Can you work these out from the model? Positions are in its coordinate system, mm. A direction names the side the tool comes from. Round coordinates to 2 decimals unless told otherwise and drop trailing zeros. Write each loop counter-clockwise with the first axis right and the second up, starting at its lowest first coordinate (ties: lowest second). Pieces come first, ordered by that corner, then holes. Notation, with made-up numbers: (2.5, -35.5) -> (53.5, -35.5) arc R37 cw to (53.5, 0.5) -> close; hole circle Ø6 at (73, 14). An arc over 180 degrees is marked (long way). Write item = value, one per line. Start each with the question number.
1) Imagine slicing it at C-C, the plane y = 12.25. Please give me the cut outline in (x, z), then the cut area to 3 significant figures.
2) Thinking about a two-plate mould opening in X: for faces 4 (the face through (25, 1, -17)), 5 (the face through (-12.97, 10.39, -18.84)), 6 (the face through (0, 3, 20)), 7 (the face through (-25, 1, -17)), which applies, +X half, -X half, draft (parallel to the pull), parting line (faces both ways), or undercut?
3) For faces 1 (the face through (20, 1, -12)), 2 (the face through (0, 1, 18)), 3 (the face through (-20, 1, 12)), which set-ups out of +Z, -Z, +X, -X, +Y, -Y let a thin tool reach every point of the face, with its end or its side?
4) If I drill on line 1 (X direction, y = 1.6, z = 16.5); line 2 (X direction, y = 0.75, z = -16.5); line 3 (X direction, y = 2.5, z = -11), over which ranges is the centre line in solid material (lowest first)?
5) I'm going to push flat-ended pins straight in: pin 1 (7 mm diameter, centred on x = -1, z = -15, fed in from +Y); pin 2 (2 mm diameter, centred on y = 5.5, z = 1, fed in from -X); pin 3 (5.5 mm diameter, centred on y = 15, z = 12, fed in from +X). Where does each tip first touch, or does it pass through?
6) Imagine slicing it at B-B, the plane z = -7.5. Please give me the cut outline in (x, y).
7) Imagine slicing it at D-D, the plane x = 14. Please give me the cut outline in (y, z).
8) Imagine slicing it at A-A, the plane x = -20. Please give me the cut outline in (y, z), then the cut area to 3 significant figures.
from build123d import *

# Parameters (mm, degrees)
ESBO_O1_W                  = 30
ESBO_O1_H                  = 50
ESBO_O1_W_2                = 22
ESBO_O1_H_2                = 42
RESSALTO_EXTRUS_O1_DEPTH   = 20
ESBO_O3_R                  = 1.75
CORTE_EXTRUS_O2_DEPTH      = 44.874821937
CORTE_EXTRUS_O3_DEPTH      = 44.874821937
CORTE_EXTRUS_O3_DEPTH_BACK = 44.874821937
ESBO_O6_R                  = 1.75
ESBO_O6_W                  = 50
ESBO_O6_H                  = 9
RESSALTO_EXTRUS_O2_DEPTH   = 3


with BuildPart() as part:
    # Esbo_o1 → Ressalto-extrus_o1 (new body)
    with BuildSketch(Plane(origin=(0, 0, 0), x_dir=(1, 0, 0), z_dir=(0, 1, 0))):
        Rectangle(ESBO_O1_W, ESBO_O1_H)
        Rectangle(ESBO_O1_W_2, ESBO_O1_H_2, mode=Mode.SUBTRACT)
    extrude(amount=RESSALTO_EXTRUS_O1_DEPTH)

    # Esbo_o3 → Corte-extrus_o2 (cut, through all)
    with BuildSketch(Plane(origin=(15, 0, 0), x_dir=(0, 0, -1), z_dir=(1, 0, 0))):
        with Locations((-12, 15)):
            Circle(ESBO_O3_R)
        with Locations((12, 15)):
            Circle(ESBO_O3_R)
    extrude(amount=-CORTE_EXTRUS_O2_DEPTH, mode=Mode.SUBTRACT)

    # Esbo_o5 → Corte-extrus_o3 (cut, two sides: drawn at the far end of the back side and taken through both)
    with BuildSketch(Plane.ZY.offset(15).offset(-CORTE_EXTRUS_O3_DEPTH_BACK)):
        with BuildLine():
            Line((-16.736274298, 16.602406244), (-21, 4))
            Line((-21, 4), (-21, 0))
            Line((-21, 0), (-25, 0))
            Line((-25, 0), (-25, 4))
            Line((-25, 4), (-25, 20))
            Line((-25, 20), (-12, 20))
            ThreePointArc((-12, 20), (-14.914444096, 19.062759605), (-16.736274298, 16.602406244))
        make_face()
        with BuildLine():
            Line((25, 0), (25, 4))
            Line((25, 4), (25, 20))
            Line((25, 20), (12, 20))
            ThreePointArc((12, 20), (14.914444096, 19.062759605), (16.736274298, 16.602406244))
            Line((16.736274298, 16.602406244), (21, 4))
            Line((21, 4), (21, 0))
            Line((21, 0), (25, 0))
        make_face()
    extrude(amount=CORTE_EXTRUS_O3_DEPTH + CORTE_EXTRUS_O3_DEPTH_BACK, mode=Mode.SUBTRACT)


with BuildPart() as corte_extrus_o3_piece_1:
    # of the separate pieces the step leaves, piece 1, a body of its own (corte_extrus_o3_pieces)
    add(part.part.solids().sort_by_distance((-15, 0, 21))[0])



with BuildPart() as corte_extrus_o3_piece_2:
    # of the separate pieces the step leaves, piece 2, a body of its own (corte_extrus_o3_pieces)
    add(part.part.solids().sort_by_distance((15, 0, -21))[0])


with BuildPart() as corte_extrus_o3_piece_1_1:
    add(corte_extrus_o3_piece_1.part)

    add(corte_extrus_o3_piece_2.part)  # Ressalto-extrus_o2 merges Corte-extrus_o3 piece 2
    # Esbo_o6 → Ressalto-extrus_o2 (add)
    # profile 1 of 2: a face of its own
    with BuildSketch(Plane.XZ):
        Polygon((-15, 21), (15, 21), (25, 21), (25, 12), (15, 12), (15, 18), (-15, 18), (-15, 12), (-25, 12), (-25, 21), align=None)
        with Locations(Location((20, 16.5, 0), (0, 0, 90))):
            Circle(ESBO_O6_R, mode=Mode.SUBTRACT)
        with Locations(Location((-20, 16.5, 0), (0, 0, 90))):
            Circle(ESBO_O6_R, mode=Mode.SUBTRACT)
    # profile 2 of 2: a face of its own
    with BuildSketch(Plane.XZ):
        with Locations((0, -16.5)):
            Rectangle(ESBO_O6_W, ESBO_O6_H)
        with Locations(Location((-20, -16.5, 0), (0, 0, 270))):
            Circle(ESBO_O6_R, mode=Mode.SUBTRACT)
        with Locations(Location((20, -16.5, 0), (0, 0, 270))):
            Circle(ESBO_O6_R, mode=Mode.SUBTRACT)
    extrude(amount=-RESSALTO_EXTRUS_O2_DEPTH)


solid = corte_extrus_o3_piece_1_1.part
Reported:
q1.outline = (-15, -18.21) -> (-11, -18.21) -> (-11, 18.21) -> (-15, 18.21) -> close; (11, -18.21) -> (15, -18.21) -> (15, 18.21) -> (11, 18.21) -> close
q1.area = 291 mm²
q2.face_4 = +X half
q2.face_5 = draft
q2.face_6 = undercut
q2.face_7 = -X half
q3.face_1 = +X, +Y, -Y
q3.face_2 = +Y, -Y
q3.face_3 = -X, +Y, -Y
q4.line_1 = -25 to -21.75, -18.25 to -11, 11 to 18.25, 21.75 to 25
q4.line_2 = -25 to -21.75, -18.25 to 18.25, 21.75 to 25
q4.line_3 = -15 to -11, 11 to 15
q5.pin_1 = 3
q5.pin_2 = -15
q5.pin_3 = 15
q6.outline = (-15, 0) -> (-11, 0) -> (-11, 20) -> (-15, 20) -> close; (11, 0) -> (15, 0) -> (15, 20) -> (11, 20) -> close
q7.outline = (0, -21) -> (4, -21) -> (16.6, -16.74) arc R5 ccw to (20, -12) -> (20, 12) arc R5 ccw to (16.6, 16.74) -> (4, 21) -> (0, 21) -> close; hole circle Ø3.5 at (15, -12); hole circle Ø3.5 at (15, 12)
q8.outline = (0, -21) -> (3, -21) -> (3, -18.25) -> (0, -18.25) -> close; (0, -14.75) -> (3, -14.75) -> (3, -12) -> (0, -12) -> close; (0, 12) -> (3, 12) -> (3, 14.75) -> (0, 14.75) -> close; (0, 18.25) -> (3, 18.25) -> (3, 21) -> (0, 21) -> close
q8.area = 33.0 mm²
